Source: CAD feature listing. Evaluate the final solid. Frame: model axes, mm. Face numbers are marked on the shaded views. A direction names the side the tool comes from. Coordinates: 2 decimals unless noted, no trailing zeros. Order: outer loops, then holes, each group sorted by start corner. A loop starts at its lowest first (then second) coordinate and runs counter-clockwise, first axis right, second up.
```python
from build123d import *

# Parameters (mm, degrees)
SKETCH_1_W               = 28
SKETCH_1_H               = 64
EXTRUDE_1_DEPTH          = 74
SKETCH_2_R               = 2.5
CUT_EXTRUDE_1_DEPTH      = 10
CUT_EXTRUDE_2_DEPTH      = 99.833192805
CUT_EXTRUDE_2_DEPTH_BACK = 99.833192805
SKETCH_3_W               = 54
SKETCH_3_H               = 40
EXTRUDE_2_DEPTH          = 80
SKETCH_6_R               = 10.5
CUT_EXTRUDE_3_DEPTH      = 123.719191653
SKETCH_11_W              = 28
SKETCH_11_H              = 5
SKETCH_11_H_2            = 4
EXTRUDE_5_DEPTH          = 67
SKETCH_12_R              = 2
CUT_EXTRUDE_8_DEPTH      = 122.231184107
CHAMFER_1_SIZE           = 10
SKETCH_13_R              = 10.5
SKETCH_13_R_2            = 9.5
EXTRUDE_6_DEPTH          = 25
SKETCH_14_R              = 2
CUT_EXTRUDE_9_DEPTH      = 119.894911582
SKETCH_15_R              = 2
CUT_EXTRUDE_10_DEPTH     = 122.342490596
CHAMFER_2_SIZE           = 3


with BuildPart() as part:
    # 草图1 → 凸台-拉伸1 (new body)
    with BuildSketch(Plane.XY):
        with Locations((0, 32)):
            Rectangle(SKETCH_1_W, SKETCH_1_H)
    extrude(amount=EXTRUDE_1_DEPTH)

    # 草图2 → 切除-拉伸1 (cut)
    with BuildSketch(Plane.XY.offset(74)):
        with Locations((-8, 58)):
            Circle(SKETCH_2_R)
        with Locations((8, 58)):
            Circle(SKETCH_2_R)
        with Locations((-8, 6)):
            Circle(SKETCH_2_R)
        with Locations((8, 6)):
            Circle(SKETCH_2_R)
    extrude(amount=-CUT_EXTRUDE_1_DEPTH, mode=Mode.SUBTRACT)

    # 草图3 → 切除-拉伸2 (cut, two sides: drawn at the far end of the back side and taken through both)
    with BuildSketch(Plane(origin=(0, 0, 0), x_dir=(0, 0, -1), z_dir=(1, 0, 0)).offset(-CUT_EXTRUDE_2_DEPTH_BACK)):
        with Locations((-37, 32)):
            Rectangle(SKETCH_3_W, SKETCH_3_H)
    extrude(amount=CUT_EXTRUDE_2_DEPTH + CUT_EXTRUDE_2_DEPTH_BACK, mode=Mode.SUBTRACT)

    # 草图4 → 凸台-拉伸2 (add)
    with BuildSketch(Plane(origin=(0, 0, 42), x_dir=(-1, 0, 0), z_dir=(0, 0, -1))):
        with BuildLine():
            Line((-14, 2), (14, 2))
            Line((14, 2), (14, -14))
            ThreePointArc((14, -14), (0, -28), (-14, -14))
            Line((-14, -14), (-14, 2))
        make_face()
        with BuildLine():
            Line((14, 62), (14, 78))
            ThreePointArc((14, 78), (0, 92), (-14, 78))
            Line((-14, 78), (-14, 62))
            Line((-14, 62), (14, 62))
        make_face()
    extrude(amount=EXTRUDE_2_DEPTH)

    # 草图6 → 切除-拉伸3 (cut, through all)
    with BuildSketch(Plane(origin=(0, 0, 42), x_dir=(-1, 0, 0), z_dir=(0, 0, -1))):
        with Locations((0, -14)):
            Circle(SKETCH_6_R)
        with Locations(Location((0, 78, 0), (0, 0, 180))):
            Circle(SKETCH_6_R)
    extrude(amount=CUT_EXTRUDE_3_DEPTH, mode=Mode.SUBTRACT)

    # 草图11 → 凸台-拉伸5 (add)
    with BuildSketch(Plane(origin=(0, 0, 0), x_dir=(-1, 0, 0), z_dir=(0, 0, -1))):
        with Locations((0, 64.5)):
            Rectangle(SKETCH_11_W, SKETCH_11_H)
        Rectangle(SKETCH_11_W, SKETCH_11_H_2)
    extrude(amount=EXTRUDE_5_DEPTH)

    # 草图12 → 切除-拉伸8 (cut, through all)
    with BuildSketch(Plane(origin=(0, 67, 0), x_dir=(1, 0, 0), z_dir=(0, 1, 0))):
        with Locations(Location((-9, 62, 0), (0, 0, 270))):
            Circle(SKETCH_12_R)
        with Locations(Location((9, 62, 0), (0, 0, 270))):
            Circle(SKETCH_12_R)
    extrude(amount=-CUT_EXTRUDE_8_DEPTH, mode=Mode.SUBTRACT)

    # 倒角1
    chamfer_1_edges = [part.edges().sort_by_distance(p)[0] for p in [
        (0, 62, 0),
        (0, 2, 0),
    ]]
    chamfer(chamfer_1_edges, length=CHAMFER_1_SIZE)

    # 草图13 → 凸台-拉伸6 (add, symmetric)
    # profile 1 of 2: a face of its own
    with BuildSketch(Plane.XY.offset(2)):
        with Locations((0, 78)):
            Circle(SKETCH_13_R)
        with Locations((0, 78)):
            Circle(SKETCH_13_R_2, mode=Mode.SUBTRACT)
    # profile 2 of 2: a face of its own
    with BuildSketch(Plane.XY.offset(2)):
        with Locations(Location((0, -14, 0), (0, 0, 180))):
            Circle(SKETCH_13_R)
        with Locations(Location((0, -14, 0), (0, 0, 180))):
            Circle(SKETCH_13_R_2, mode=Mode.SUBTRACT)
    extrude(amount=EXTRUDE_6_DEPTH, both=True)

    # 草图14 → 切除-拉伸9 (cut, through all)
    with BuildSketch(Plane(origin=(0, 0, 0), x_dir=(0, 0, -1), z_dir=(1, 0, 0))):
        with Locations((-34, 78)):
            Circle(SKETCH_14_R)
        with Locations((30, 78)):
            Circle(SKETCH_14_R)
        with Locations((30, -14)):
            Circle(SKETCH_14_R)
        with Locations((-34, -14)):
            Circle(SKETCH_14_R)
    extrude(amount=-CUT_EXTRUDE_9_DEPTH, mode=Mode.SUBTRACT)

    # 草图15 → 切除-拉伸10 (cut, through all)
    with BuildSketch(Plane.ZY.offset(14)):
        with Locations(Location((44, 58, 0), (0, 0, 270))):
            Circle(SKETCH_15_R)
    extrude(amount=-CUT_EXTRUDE_10_DEPTH, mode=Mode.SUBTRACT)

    # 倒角2
    chamfer_2_edges = [part.edges().sort_by_distance(p)[0] for p in [
        (-9, -2, -64),
        (-9, 67, -64),
        (9, -2, -64),
        (9, 67, -64),
    ]]
    chamfer(chamfer_2_edges, length=CHAMFER_2_SIZE - 0.0001)  # a hair under: the kernel refuses the full size


solid = part.part
```
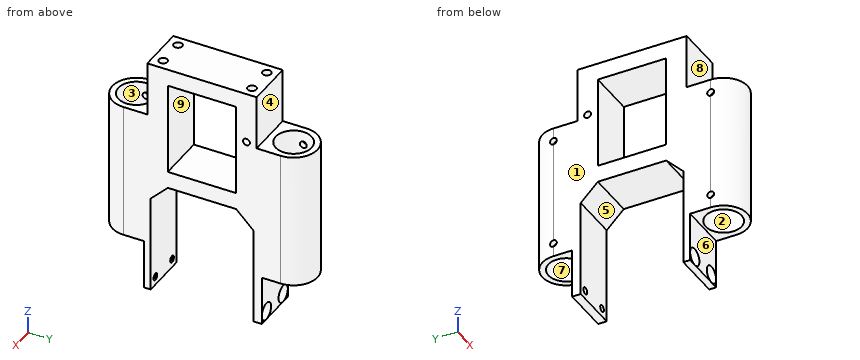
1. Section query B-B, the plane y = 45.5. Output: boundary loops of the cut face in (x, z), plus the area to 3 significant figures.
2. Material intervals for line 1 along Z through (x, y) = (-13.05, -14); line 2 along Y through (x, z) = (-8, 69.5); line 3 along Y through (x, z) = (0, -30.5), sorted ascending.
3. Draft query along X for the marked faces 1, 2, 3 and 4. Return one class per face: +X half, -X half, draft (parallel to the pull), parting line (faces both ways), or undercut.
4. Section query A-A, the plane z = 44. Output: boundary loops of the cut face in (x, y), plus the area to 3 significant figures.
5. Section query C-C, the plane z = -62. Count the separate pieces of the cut face and the enclosed holes in it, plus the area to 3 significant figures.
6. Access query for the marked faces 5, 6, 7, 8 and 9. Directions: +Z, -Z, +X, -X, +Y, -Y. A direction counts if a zero-diameter tool reaches every point of the face in a straight line with its end or side. Return the directions, or none.
7. Section query D-D, the plane y = 6. Output: boundary loops of the cut face in (x, z).
8. Contact query for flat-ended pins moving along their axis: P1, Ø6.5, axis at x = 8, y = 58, coming from the -Z side; P2, Ø2.5, axis at y = 78, z = 34, coming from the -X side; P3, Ø1.5, axis at x = -8, z = 27.5, coming from the -Y side. Output: stop coordinate, or through.
Answer key:
1. outline: (-14, 0) - (14, 0) - (14, 10) - (-14, 10) - close; (-14, 64) - (14, 64) - (14, 74) - (-14, 74) - close
1. area: 560 mm2
2. line 1: z = -38 to -32, -28 to 32, 36 to 42
2. line 2: y = 0 to 3.5, 8.5 to 55.5, 60.5 to 64
2. line 3: y = -28 to -24.5, -3.5 to 2, 62 to 67.5, 88.5 to 92
3. face 1: -X half
3. face 2: undercut
3. face 3: undercut
3. face 4: draft
4. outline: (-14, 0) - (14, 0) - (14, 12) - (-14, 12) - close; (-14, 52) - (14, 52) - (14, 56) - (-14, 56) - close; (-14, 60) - (14, 60) - (14, 64) - (-14, 64) - close
4. area: 560 mm2
5. separate pieces: 6
5. enclosed holes: 0
5. area: 144 mm2
6. face 5: -Z, +X, -X
6. face 6: -Z, +X, -X, -Y
6. face 7: -Z
6. face 8: +Z, +X, -X, -Y
6. face 9: +X, -X
7. outline: (-14, -6) - (14, -6) - (14, 74) - (10.5, 74) - (10.5, 64) - (5.5, 64) - (5.5, 74) - (-5.5, 74) - (-5.5, 64) - (-10.5, 64) - (-10.5, 74) - (-14, 74) - close
8. P1: stops at z = -9.25
8. P2: stops at x = 10.43
8. P3: stops at y = -25.98
